```python
from build123d import *

# Parameters (mm, degrees)
F0_W     = 570
F0_H     = 550
F0_R     = 1.5
F0_W_2   = 370
F0_H_2   = 400
F1_DEPTH = 2.5


with BuildPart() as f1:
    # F0 (on Front) → F1 (new body, symmetric)
    with BuildSketch(Plane.XZ):
        Rectangle(F0_W, F0_H)
        with Locations((-271, -268)):
            Circle(F0_R, mode=Mode.SUBTRACT)
        with Locations((-253, -268)):
            Circle(F0_R, mode=Mode.SUBTRACT)
        with Locations((-271, -251)):
            Circle(F0_R, mode=Mode.SUBTRACT)
        with Locations((253, -268)):
            Circle(F0_R, mode=Mode.SUBTRACT)
        with Locations((271, -268)):
            Circle(F0_R, mode=Mode.SUBTRACT)
        with Locations((271, -251)):
            Circle(F0_R, mode=Mode.SUBTRACT)
        with Locations((-272, 252)):
            Circle(F0_R, mode=Mode.SUBTRACT)
        with Locations((-262, 262)):
            Circle(F0_R, mode=Mode.SUBTRACT)
        Rectangle(F0_W_2, F0_H_2, mode=Mode.SUBTRACT)
        with Locations((272, 252)):
            Circle(F0_R, mode=Mode.SUBTRACT)
        with Locations((262, 262)):
            Circle(F0_R, mode=Mode.SUBTRACT)
    extrude(amount=F1_DEPTH, both=True)


solid = f1.part
```
The listing builds one solid part. Answer for the finished solid, in the listing's coordinates (mm). Give positions to 0.01 mm unless a question says otherwise; leave off trailing zeros. Order: outer loops, then holes, each group sorted by start corner. A loop starts at its lowest first (then second) coordinate and runs counter-clockwise, first axis right, second up. Notation, with made-up numbers: M 21,42 L 59,42 A16 cw 59,62 Z; hole C 55.5,-40 d5. An arc over 180 degrees is marked long. Put each result on its own line as item: value. Start each with the question number.
Item 1: Find the intervals of material crossed by line 1 along X through (y, z) = (0, 262); line 2 along X through (y, z) = (-0.4, 252); line 3 along X through (y, z) = (0.1, -268), in increasing order.
Item 2: The part is cut by section A-A, the plane z = 68. Determine the outline of the cut face in (x, y), and give its area (3 significant figures).
Item 3: The part is cut by section B-B, the plane x = 126.5. Determine the outline of the cut face in (y, z), and give its area (3 significant figures).
Item 4: The part is cut by section C-C, the plane y = 0.2. State how many separate pieces and enclosed holes the cut face has, and give its area (3 significant figures).
Answer key:
1. line 1: x = -285 to -263.5, -260.5 to 260.5, 263.5 to 285
1. line 2: x = -285 to -273.5, -270.5 to 270.5, 273.5 to 285
1. line 3: x = -285 to -272.5, -269.5 to -254.5, -251.5 to 251.5, 254.5 to 269.5, 272.5 to 285
2. outline: M -285,-2.5 L -185,-2.5 L -185,2.5 L -285,2.5 Z; M 185,-2.5 L 285,-2.5 L 285,2.5 L 185,2.5 Z
2. area: 1,000 mm²
3. outline: M -2.5,-275 L 2.5,-275 L 2.5,-200 L -2.5,-200 Z; M -2.5,200 L 2.5,200 L 2.5,275 L -2.5,275 Z
3. area: 750 mm²
4. separate pieces: 1
4. enclosed holes: 11
4. area: 165,000 mm²
